Geometry check sheet. Reference: the model listing, model coordinates, mm. A direction names the side the tool comes from. Round coordinates to 2 decimals unless told otherwise and drop trailing zeros. Write each loop counter-clockwise with the first axis right and the second up, starting at its lowest first coordinate (ties: lowest second). Pieces come first, ordered by that corner, then holes. Notation, with made-up numbers: M 46.25,73 L 87.25,73 A6 ccw 87.25,82 Z; hole C -27,76 d9. An arc over 180 degrees is marked long. Use a Markdown table: item, result.
```python
from build123d import *

# Parameters (mm, degrees)
SKETCH1_W             = 50.8
SKETCH1_H             = 34.036
BOSS_EXTRUDE1_DEPTH   = 1.5875
SKETCH2_W             = 50.8
SKETCH2_H             = 3.175
BOSS_EXTRUDE2_DEPTH   = 19.05
CHAMFER1_SIZE         = 12.7
F_3_0MM_DOWEL_HOLE1_D = 3
CHAMFER2_SIZE         = 3.175
CUT_EXTRUDE1_DEPTH    = 3.175
SKETCH7_R             = 8.255
CUT_EXTRUDE3_DEPTH    = 3.175
SKETCH8_R             = 8.255
CUT_EXTRUDE4_DEPTH    = 3.175
SKETCH9_R             = 0.8
CUT_EXTRUDE5_DEPTH    = 3.175
CUT_EXTRUDE6_DEPTH    = 3.175
SKETCH13_R            = 2.5
SKETCH13_R_2          = 1.5
CUT_EXTRUDE7_DEPTH    = 45.982971525


with BuildPart() as part:
    # Sketch1 → Boss-Extrude1 (new, symmetric)
    with BuildSketch(Plane.XY):
        Rectangle(SKETCH1_W, SKETCH1_H)
    extrude(amount=BOSS_EXTRUDE1_DEPTH, both=True)

    # Sketch2 → Boss-Extrude2 (add)
    with BuildSketch(Plane.XY.offset(1.5875)):
        with Locations((0, -15.4305)):
            Rectangle(SKETCH2_W, SKETCH2_H)
    extrude(amount=BOSS_EXTRUDE2_DEPTH)

    # Chamfer1
    chamfer1_edges = [part.edges().sort_by_distance(p)[0] for p in [
        (-25.4, -15.4305, 20.6375),
        (25.4, -15.4305, 20.6375),
    ]]
    chamfer(chamfer1_edges, length=CHAMFER1_SIZE)

    # Ø3.0mm Dowel Hole1 (through all)
    with Locations(Plane(origin=(0, -13.843, 0), x_dir=(1, 0, 0), z_dir=(0, 1, 0))):
        with Locations((-12.7, -14.2875), (12.7, -14.2875)):
            Hole(F_3_0MM_DOWEL_HOLE1_D / 2)

    # Chamfer2
    chamfer2_edges = [part.edges().sort_by_distance(p)[0] for p in [
        (25.4, 17.018, 0),
        (-25.4, 17.018, 0),
    ]]
    chamfer(chamfer2_edges, length=CHAMFER2_SIZE)

    # Sketch5 → Cut-Extrude1 (cut)
    with BuildSketch(Plane(origin=(0, 0, -1.5875), x_dir=(-1, 0, 0), z_dir=(0, 0, -1))):
        with BuildLine():
            Line((-5.969, 14.001104381), (-5.969, 17.018))
            Line((-5.969, 17.018), (5.969, 17.018))
            Line((5.969, 17.018), (5.969, 14.001104381))
            ThreePointArc((5.969, 14.001104381), (5.225051224, 12.205053157), (3.429, 11.461104381))
            Line((3.429, 11.461104381), (-3.429, 11.461104381))
            ThreePointArc((-3.429, 11.461104381), (-5.225051224, 12.205053157), (-5.969, 14.001104381))
        make_face()
    extrude(amount=-CUT_EXTRUDE1_DEPTH, mode=Mode.SUBTRACT)

    # Sketch7 → Cut-Extrude3 (cut)
    with BuildSketch(Plane(origin=(0, 0, -1.5875), x_dir=(-1, 0, 0), z_dir=(0, 0, -1))):
        with Locations((12.896, 6.34)):
            Circle(SKETCH7_R)
    extrude(amount=-CUT_EXTRUDE3_DEPTH, mode=Mode.SUBTRACT)

    # Sketch8 → Cut-Extrude4 (cut)
    with BuildSketch(Plane(origin=(0, 0, -1.5875), x_dir=(-1, 0, 0), z_dir=(0, 0, -1))):
        with Locations((-13.104, 6.34)):
            Circle(SKETCH8_R)
    extrude(amount=-CUT_EXTRUDE4_DEPTH, mode=Mode.SUBTRACT)

    # Sketch9 → Cut-Extrude5 (cut)
    with BuildSketch(Plane.XY.offset(1.5875)):
        with Locations((-21.306, 15.21)):
            Circle(SKETCH9_R)
        with Locations((21.514, 15.21)):
            Circle(SKETCH9_R)
        with Locations((21.514, -2.53)):
            Circle(SKETCH9_R)
        with Locations((-21.306, -2.53)):
            Circle(SKETCH9_R)
    extrude(amount=-CUT_EXTRUDE5_DEPTH, mode=Mode.SUBTRACT)

    # Sketch11 → Cut-Extrude6 (cut)
    with BuildSketch(Plane(origin=(0, -13.843, 0), x_dir=(1, 0, 0), z_dir=(0, 1, 0))):
        Polygon((-12.7, -20.6375), (-25.4, -1.5875), (-25.4, -7.9375), align=None)
        Polygon((25.4, -1.5875), (12.7, -20.6375), (25.4, -7.9375), align=None)
    extrude(amount=-CUT_EXTRUDE6_DEPTH, mode=Mode.SUBTRACT)

    # Sketch13 → Cut-Extrude7 (cut, through all)
    with BuildSketch(Plane(origin=(0, -13.843, 0), x_dir=(1, 0, 0), z_dir=(0, 1, 0))):
        with Locations(Location((0, -14.2875, 0), (0, 0, 270))):
            Circle(SKETCH13_R)
        with Locations(Location((-12.7, -14.2875, 0), (0, 0, 270))):
            Circle(SKETCH13_R_2)
        with Locations(Location((12.7, -14.2875, 0), (0, 0, 270))):
            Circle(SKETCH13_R_2)
    extrude(amount=-CUT_EXTRUDE7_DEPTH, mode=Mode.SUBTRACT)


solid = part.part
```
Item 1: Material ranges on line 1 along Z through (x, y) = (15, -5); line 2 along Y through (x, z) = (-12, 6); line 3 along Y through (x, z) = (-9, -0.5), recorded low to high. Write a range as from..to.
Outcome:
| item | result |
|---|---|
| line 1 | z = -1.59..1.59 |
| line 2 | y = -17.02..-13.84 |
| line 3 | y = -17.02..-0.94, 13.62..17.02 |
Item 2: Access from +Z, -Z, +X, -X, +Y, -Y to the whole of each face (thin tool, end or side, straight path). Record for faces 4 (the face through (5.21, 12.19, -0.02)), 5 (the face through (19.14, -15.41, 10.98)), 6 (the face through (0, -2, 1.588)).
Outcome:
| item | result |
|---|---|
| face 4 | +Z, -Z, +Y |
| face 5 | +Z, +X, +Y, -Y |
| face 6 | +Z, +X, -X, +Y |
Item 3: Mould release check, pull along Y, two halves, no side actions. Record for faces 1 (the face through (25.4, -2, 0)), 2 (the face through (-6.345, 1.317, -0.022)), 3 (the face through (23.835, 15.408, 0.022)): +Y half, -Y half, draft (parallel to the pull), parting line (faces both ways), or undercut.
Outcome:
| item | result |
|---|---|
| face 1 | draft |
| face 2 | undercut |
| face 3 | +Y half |
Item 4: Cross-section at C-C, the plane y = 15.21. Record the cut outline in (x, z).
Outcome:
| item | result |
|---|---|
| outline | M -24.03,-1.59 L -22.11,-1.59 L -22.11,1.59 L -24.03,1.59 Z; M -20.51,-1.59 L -5.97,-1.59 L -5.97,1.59 L -20.51,1.59 Z; M 5.97,-1.59 L 20.71,-1.59 L 20.71,1.59 L 5.97,1.59 Z; M 22.31,-1.59 L 24.03,-1.59 L 24.03,1.59 L 22.31,1.59 Z |
Item 5: Go/stop test with flat-tipped pins: pin 1 (1.5 mm diameter, centred on y = 15.5, z = -0.5, fed in from -X); pin 2 (1.8 mm diameter, centred on x = 21.514, y = -2.53, fed in from +Z); pin 3 (12 mm diameter, centred on y = -11.5, z = 16, fed in from +X). Record where each tip stops, or that it passes through.
Outcome:
| item | result |
|---|---|
| pin 1 | stops at x = -24.49 |
| pin 2 | stops at z = 1.59 |
| pin 3 | stops at x = 19.47 |
Item 6: Cross-section at D-D, the plane x = 9.5. Record the cut outline in (y, z).
Outcome:
| item | result |
|---|---|
| outline | M -17.02,-1.59 L -1.09,-1.59 L -1.09,1.59 L -13.84,1.59 L -13.84,20.64 L -17.02,20.64 Z; M 13.77,-1.59 L 17.02,-1.59 L 17.02,1.59 L 13.77,1.59 Z |
Item 7: Cross-section at A-A, the plane x = 0. Record the cut outline in (y, z), and give its area (3 significant figures).
Outcome:
| item | result |
|---|---|
| outline | M -17.02,-1.59 L 11.46,-1.59 L 11.46,1.59 L -13.84,1.59 L -13.84,11.79 L -17.02,11.79 Z; M -17.02,16.79 L -13.84,16.79 L -13.84,20.64 L -17.02,20.64 Z |
| area | 135 mm2 |
Item 8: Cross-section at B-B, the plane y = -2.53. Record the cut outline in (x, z).
Outcome:
| item | result |
|---|---|
| outline | M -25.4,-1.59 L -22.11,-1.59 L -22.11,1.59 L -25.4,1.59 Z; M -20.51,-1.59 L 20.71,-1.59 L 20.71,1.59 L -20.51,1.59 Z; M 22.31,-1.59 L 25.4,-1.59 L 25.4,1.59 L 22.31,1.59 Z |
